Check sheet for the modelled part. Datum: model origin and axes. Units: mm. A direction names the side the tool comes from. Give positions to 0.01 mm unless a question says otherwise; leave off trailing zeros. Order: outer loops, then holes, each group sorted by start corner. A loop starts at its lowest first (then second) coordinate and runs counter-clockwise, first axis right, second up. Notation, with made-up numbers: (-20.75, 21.25) -> (1.25, 21.25) arc R15 cw to (1.25, 48.25) -> close; hole circle Ø11 at (80, 68). An arc over 180 degrees is marked (long way). Answer in a Markdown table with one row per item. Add a question column.
(1) Release check for a two-part mould opening along Y. For faces 1 (the face through (0, 0, 12)), 2 (the face through (3.22, 14.52, 0.87)), 3 (the face through (0, 6, 0)) record: released by +Y, released by -Y, zero draft, split by the parting line, or undercut.
(2) Set-up check for faces 4 (the face through (14, 0, 19)), 5 (the face through (1.08, 4.88, 5.88)), 6 (the face through (-10.635, -3.349, 15.549)): record each of +Z, -Z, +X, -X, +Y, -Y from which the full face is reachable in a straight line by a thin tool's end or side.
(3) Cross-section at C-C (z = 2). Record the cut outline in (x, y).
(4) Thickness scan on L1, parallel to Y at x = 0, z = 6.75; L2, parallel to X at y = 7.5, z = 13.25; L3, parallel to Y at x = 0, z = 14.5. Record the ranges inside material, lowest first. Write a range as [from, to].
(5) Go/stop test with flat-tipped pins: pin 1 (18 mm diameter, centred on x = -1.5, y = -1, fed in from +Z); pin 2 (10 mm diameter, centred on x = -9.5, y = -14.5, fed in from -Z); pin 3 (3 mm diameter, centred on x = -18.5, z = 15, fed in from -Y); pin 4 (12 mm diameter, centred on x = -15.5, y = -24, fed in from -Z). Record where each tip stops, or that it passes through.
(6) Cross-section at A-A (y = 0). Record the cut outline in (x, z), then the cut area to 3 significant figures.
(7) Cross-section at D-D (z = 14). Record the cut outline in (x, y), then the cut area to 3 significant figures.
```python
from build123d import *

# Parameters (mm, degrees)
F0_W     = 5
F0_H     = 0.4
F2_R     = 32
F3_DEPTH = 25


with BuildPart() as f1:
    # F0 (on Front) → F1 (revolve)
    with BuildSketch(Plane.XZ):
        Polygon((-14, 0), (-5, 0), (-5, 11.6), (-5, 12), (-11.15, 12), (-11.15, 19), (-33, 19), align=None)
        with Locations((-2.5, 11.8)):
            Rectangle(F0_W, F0_H)
    revolve(axis=Axis((0, 0, 11.8), (0, 0, 1)))


with BuildPart() as f3:
    # F2 (on Top) → F3 (new body)
    with BuildSketch(Plane.XY):
        Circle(F2_R)
    extrude(amount=F3_DEPTH)


with BuildPart() as f1_1:
    add(f1.part)

    # F4: intersect F3
    add(f3.part, mode=Mode.INTERSECT)


solid = f1_1.part
```
Answer below:
| question | item | result |
|---|---|---|
| 1 | face 1 | undercut |
| 1 | face 2 | split by the parting line |
| 1 | face 3 | zero draft |
| 2 | face 4 | +Z, +X, -X, +Y, -Y |
| 2 | face 5 | -Z |
| 2 | face 6 | +Z |
| 3 | outline | circle Ø32 at (0, 0); hole circle Ø10 at (0, 0) |
| 4 | L1 | y = [-20.75, -5], [5, 20.75] |
| 4 | L2 | x = [-26.2, -8.25], [8.25, 26.2] |
| 4 | L3 | y = [-28.5, -11.15], [11.15, 28.5] |
| 5 | pin 1 | stops at z = 12 |
| 5 | pin 2 | stops at z = 0 |
| 5 | pin 3 | stops at y = -24.56 |
| 5 | pin 4 | stops at z = 8.57 |
| 6 | outline | (-32, 18) -> (-14, 0) -> (-5, 0) -> (-5, 11.6) -> (5, 11.6) -> (5, 0) -> (14, 0) -> (32, 18) -> (32, 19) -> (11.15, 19) -> (11.15, 12) -> (-11.15, 12) -> (-11.15, 19) -> (-32, 19) -> close |
| 6 | area | 620 mm² |
| 7 | outline | circle Ø56 at (0, 0); hole circle Ø22.3 at (0, 0) |
| 7 | area | 2,070 mm² |
